```python
from build123d import *

# Parameters (mm, degrees)
SKETCH1_W           = 38.1
SKETCH1_H           = 25.4
BOSS_EXTRUDE1_DEPTH = 3.175
SKETCH2_W           = 25.4
SKETCH2_H           = 25.4
BOSS_EXTRUDE2_DEPTH = 6.35
CUT_EXTRUDE1_REACH  = 34.379
SKETCH3_W           = 3.175
SKETCH3_H           = 3.175
SKETCH3_W_2         = 6.35
SKETCH3_H_2         = 6.35
CUT_EXTRUDE2_REACH  = 34.379
FILLET1_R           = 1.27
BOSS_EXTRUDE3_DEPTH = 19.05
CUT_EXTRUDE3_REACH  = 38.418
SKETCH6_R           = 6.35


with BuildPart() as part:
    # Sketch1 → Boss-Extrude1 (new body)
    with BuildSketch(Plane.XY):
        Rectangle(SKETCH1_W, SKETCH1_H)
    extrude(amount=BOSS_EXTRUDE1_DEPTH)

    # Sketch2 → Boss-Extrude2 (add)
    with BuildSketch(Plane(origin=(0, 0, 0), x_dir=(-1, 0, 0), z_dir=(0, 0, -1))):
        Rectangle(SKETCH2_W, SKETCH2_H)
    extrude(amount=BOSS_EXTRUDE2_DEPTH)

    # Sketch3 → Cut-Extrude1 (cut, up to next)
    with BuildSketch(Plane(origin=(0, 12.7, 0), x_dir=(1, 0, 0), z_dir=(0, 1, 0)), mode=Mode.PRIVATE) as cut_extrude1_sk1:
        with Locations((11.1125, 1.5875)):
            Rectangle(SKETCH3_W, SKETCH3_H)
    cut_extrude1_tool1 = extrude(cut_extrude1_sk1.sketch, amount=-CUT_EXTRUDE1_REACH, mode=Mode.PRIVATE) & part.part
    # Sketch3 → Cut-Extrude1 (cut, up to next)
    with BuildSketch(Plane(origin=(0, 12.7, 0), x_dir=(1, 0, 0), z_dir=(0, 1, 0)), mode=Mode.PRIVATE) as cut_extrude1_sk2:
        with Locations((3.175, 3.175)):
            Rectangle(SKETCH3_W_2, SKETCH3_H_2)
    cut_extrude1_tool2 = extrude(cut_extrude1_sk2.sketch, amount=-CUT_EXTRUDE1_REACH, mode=Mode.PRIVATE) & part.part
    cut_extrude1_1 = cut_extrude1_tool1.solids().sort_by_distance((11.1125, 12.7, -1.5875))[0]
    add(cut_extrude1_1, mode=Mode.SUBTRACT)
    cut_extrude1_2 = cut_extrude1_tool2.solids().sort_by_distance((3.175, 12.7, -3.175))[0]
    add(cut_extrude1_2, mode=Mode.SUBTRACT)
    cut_extrude1 = cut_extrude1_1 + cut_extrude1_2  # Cut-Extrude1 as one shape, for the pattern or mirror that repeats it

    # Sketch4 → Cut-Extrude2 (cut, up to next)
    with BuildSketch(Plane(origin=(0, 12.7, 0), x_dir=(1, 0, 0), z_dir=(0, 1, 0)), mode=Mode.PRIVATE) as cut_extrude2_sk1:
        Polygon((6.604, 0), (6.35, 0), (6.35, 6.35), (12.7, 6.35), (12.7, 3.175), (9.525, 3.175), (9.525, 0), (9.271, 0), (9.271, 3.429), (12.446, 3.429), (12.446, 6.096), (6.604, 6.096), align=None)
    cut_extrude2_tool1 = extrude(cut_extrude2_sk1.sketch, amount=-CUT_EXTRUDE2_REACH, mode=Mode.PRIVATE) & part.part
    cut_extrude2 = cut_extrude2_tool1.solids().sort_by_distance((6.477, 12.7, -0.089803))[0]
    add(cut_extrude2, mode=Mode.SUBTRACT)

    # Mirror1: Cut-Extrude1, Cut-Extrude2 across plane
    add(cut_extrude1.mirror(Plane.ZY), mode=Mode.SUBTRACT)
    add(cut_extrude2.mirror(Plane.ZY), mode=Mode.SUBTRACT)

    # Fillet1
    fillet1_edges = [part.edges().sort_by_distance(p)[0] for p in [
        (-6.604, 0, -6.096),
        (-12.446, 0, -6.096),
        (-12.446, 0, -3.429),
        (12.446, 0, -3.429),
        (12.446, 0, -6.096),
        (6.604, 0, -6.096),
    ]]
    fillet(fillet1_edges, radius=FILLET1_R)

    # Sketch5 → Boss-Extrude3 (add)
    with BuildSketch(Plane.XY.offset(3.175)):
        with BuildLine():
            Line((7.9375, 0), (7.9375, -12.7))
            Line((7.9375, -12.7), (-7.9375, -12.7))
            Line((-7.9375, -12.7), (-7.9375, 0))
            ThreePointArc((-7.9375, 0), (0, 7.9375), (7.9375, 0))
        make_face()
    extrude(amount=BOSS_EXTRUDE3_DEPTH)

    # Sketch6 → Cut-Extrude3 (cut, up to next)
    with BuildSketch(Plane.XY.offset(22.225), mode=Mode.PRIVATE) as cut_extrude3_sk1:
        Circle(SKETCH6_R)
    cut_extrude3_tool1 = extrude(cut_extrude3_sk1.sketch, amount=-CUT_EXTRUDE3_REACH, mode=Mode.PRIVATE) & part.part
    add(cut_extrude3_tool1.solids().sort_by_distance((0, 0, 22.225))[0], mode=Mode.SUBTRACT)


solid = part.part
```
Source: CAD feature listing. Evaluate the final solid. Frame: model axes, mm. A direction names the side the tool comes from. Round coordinates to 2 decimals unless told otherwise and drop trailing zeros. Loops run counter-clockwise (first coordinate to the right, second up) from the corner with the lowest first, then second, coordinate; pieces in that order, holes last. Notation, with made-up numbers: M 57,86.5 L 97,86.5 A23 cw 97,98.5 Z; hole C 19,-4 d9. An arc over 180 degrees is marked long. Use a Markdown table: item, result. Add a question column.
1. Pull-direction query (X, two-part tool) for faces 6 (the flat face through (-10, 0, -6.096)), 7 (the cylindrical face through (6.986, -0.178, -5.734)), 8 (the flat face through (-19.05, 0, 2)), 9 (the flat face through (6.604, 0, -2)); classes: +X half, -X half, draft (parallel to the pull), parting line (faces both ways), or undercut.
2. Set-up query: faces 1 (the flat face through (-7.938, -6, 13)), 2 (the flat face through (-14, 0, 0)), 3 (the flat face through (9.271, 0, -2)), 4 (the cylindrical face through (-0.175, 7.936, 12.567)), 5 (the flat face through (-3, 6, 0)). Return all of +Z, -Z, +X, -X, +Y, -Y with unobstructed straight access to the full face (end or side cutting, diameter ignored); none if empty.
3. Cut plane A-A, the plane z = -2.5. Output: boundary loops of the cut face in (x, y), and give its area (3 significant figures).
4. Contact query for flat-ended pins moving along their axis: pin 1 (5 mm diameter, centred on x = 14.5, y = 3.5, fed in from -Z); pin 2 (10 mm diameter, centred on y = -7, z = 11.5, fed in from -X); pin 3 (1 mm diameter, centred on x = -10.5, y = 6, fed in from +Z) (3 decimals); pin 4 (6 mm diameter, centred on x = -12, z = 7, fed in from -Y). Output: stop coordinate, or through.
5. Ray query, line 1 along Y through (x, z) = (0, 15.25); line 2 along Z through (x, y) = (9.5, -6.25) (3 decimals); line 3 along Z through (x, y) = (-14, -5.75) (3 decimals). Return the intervals inside material, ascending. Write a range as [from, to].
Solution:
| question | item | result |
|---|---|---|
| 1 | face 6 | draft |
| 1 | face 7 | undercut |
| 1 | face 8 | -X half |
| 1 | face 9 | undercut |
| 2 | face 1 | +Z, -X, +Y, -Y |
| 2 | face 2 | -X, +Y, -Y |
| 2 | face 3 | +X, +Y, -Y |
| 2 | face 4 | +Z, +Y |
| 2 | face 5 | -Z, +Y, -Y |
| 3 | outline | M -9.27,-12.7 L -6.6,-12.7 L -6.6,12.7 L -9.27,12.7 Z; M 6.6,-12.7 L 9.27,-12.7 L 9.27,12.7 L 6.6,12.7 Z |
| 3 | area | 135 mm2 |
| 4 | pin 1 | stops at z = -5.79 |
| 4 | pin 2 | stops at x = -7.94 |
| 4 | pin 3 | stops at z = 3.175 |
| 4 | pin 4 | passes through |
| 5 | line 1 | y = [-12.7, -6.35], [6.35, 7.94] |
| 5 | line 2 | z = [-6.096, -3.429], [0, 3.175] |
| 5 | line 3 | z = [0, 3.175] |
